from build123d import *

# Parameters (mm, degrees)
BOSS_EXTRUDE1_DEPTH      = 10
BOSS_EXTRUDE2_DEPTH      = 10
BOSS_EXTRUDE2_DEPTH_BACK = 20


with BuildPart() as part:
    # Sketch1 → Boss-Extrude1 (new body)
    with BuildSketch(Plane.XY):
        with BuildLine():
            Line((-125, 175), (-50, 175))
            ThreePointArc((-50, 175), (0, 125), (50, 175))
            Line((50, 175), (125, 175))
            Line((125, 175), (175, 125))
            Line((175, 125), (175, -125))
            Line((175, -125), (125, -175))
            Line((125, -175), (50, -175))
            ThreePointArc((50, -175), (0, -125), (-50, -175))
            Line((-50, -175), (-125, -175))
            Line((-125, -175), (-175, -125))
            Line((-175, -125), (-175, 125))
            Line((-175, 125), (-125, 175))
        make_face()
    extrude(amount=BOSS_EXTRUDE1_DEPTH)

    # Sketch2 → Boss-Extrude2 (add, two sides: drawn at the far end of the back side and taken through both)
    with BuildSketch(Plane.XY.offset(10).offset(-BOSS_EXTRUDE2_DEPTH_BACK)):
        Polygon((25, 125), (-2.148886373, 125), (-25, 125), (-25, 0), (-25, -125), (25, -125), align=None)
    extrude(amount=BOSS_EXTRUDE2_DEPTH + BOSS_EXTRUDE2_DEPTH_BACK)


solid = part.part
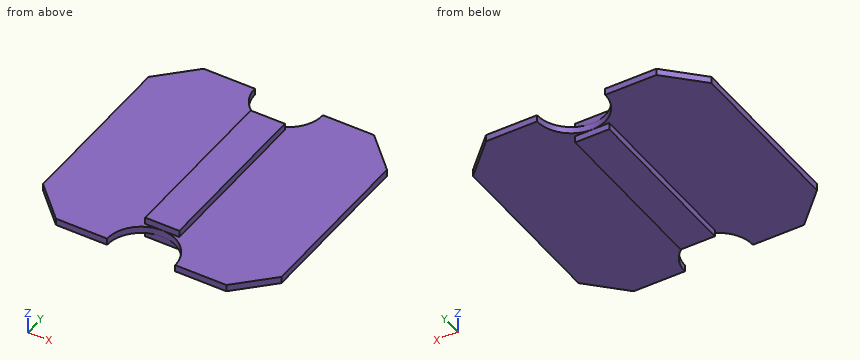
The model under review builds one solid part; all positions refer to its coordinate system, in mm. Give positions to 0.01 mm unless a question says otherwise; leave off trailing zeros. Loops run counter-clockwise (first coordinate to the right, second up) from the corner with the lowest first, then second, coordinate; pieces in that order, holes last. Notation, with made-up numbers: (54.25, 42) -> (110.25, 42) arc R14 cw to (110.25, 46) -> close; hole circle Ø2 at (-0.5, -13). An arc over 180 degrees is marked (long way). Put each result on its own line as item: value. Start each with the question number.
1. We need section B-B on y = -20. State the section outline as (x, z) points.
2. We need section A-A on y = 135. State the section outline as (x, z) points, then the cut area to 3 significant figures.
3. Clearance check with flat-ended pins moving along their axes: P1, Ø5, axis at x = -0.5, z = -6.5, coming from the -Y side; P2, Ø5, axis at y = -30, z = -4.5, coming from the -X side; P3, Ø2, axis at x = -5, z = 2, coming from the -Y side; P4, Ø2, axis at y = -111.5, z = -0.5, coming from the +X side. State where each tip first meets the part, or that it passes through.
4. We need section D-D on x = 150. State the section outline as (y, z) points, then the cut area to 3 significant figures.
5. Wall thickness on probe 1 along X at (y, z) = (30, 13.75); probe 2 along Z at (x, y) = (112, -124); probe 3 along Y at (x, z) = (-18.5, 17.5): over which ranges is each line inside the solid? List them lowest first.
6. We need section C-C on z = 5.25. State the section outline as (x, y) points.
Determined:
1. outline: (-175, 0) -> (-25, 0) -> (-25, -10) -> (25, -10) -> (25, 0) -> (175, 0) -> (175, 10) -> (25, 10) -> (25, 20) -> (-25, 20) -> (-25, 10) -> (-175, 10) -> close
2. outline: (-165, 0) -> (-30, 0) -> (-30, 10) -> (-165, 10) -> close; (30, 0) -> (165, 0) -> (165, 10) -> (30, 10) -> close
2. area: 2,700 mm^2
3. P1: y = -125
3. P2: x = -25
3. P3: y = -125.36
3. P4: x = 175
4. outline: (-150, 0) -> (150, 0) -> (150, 10) -> (-150, 10) -> close
4. area: 3,000 mm^2
5. probe 1: -25 to 25
5. probe 2: 0 to 10
5. probe 3: -125 to 125
6. outline: (-175, -125) -> (-125, -175) -> (-50, -175) arc R50 cw to (50, -175) -> (125, -175) -> (175, -125) -> (175, 125) -> (125, 175) -> (50, 175) arc R50 cw to (-50, 175) -> (-125, 175) -> (-175, 125) -> close
